Geometry check sheet. Reference: the model listing, model coordinates, mm. A direction names the side the tool comes from. Round coordinates to 2 decimals unless told otherwise and drop trailing zeros. Loops run counter-clockwise (first coordinate to the right, second up) from the corner with the lowest first, then second, coordinate; pieces in that order, holes last. Notation, with made-up numbers: (69.5, 23.5) -> (121.5, 23.5) arc R23 cw to (121.5, 44.5) -> close; hole circle Ø8 at (-21, -23). An arc over 180 degrees is marked (long way). Use a Markdown table: item, result. Add a question column.
Q1. Gauge pin test, flat ends, axial feed: P1, Ø3, axis at x = 8, z = -38, coming from the +Y side; P2, Ø0.8, axis at y = 3.5, z = 34.5, coming from the -X side. Record the tip position at first contact, or that the pin passes through.
Q2. Release check for a two-part mould opening along Y. For faces 3 (the face through (22, 0, -1)), 4 (the face through (44.034, 4.8, 37.675)), 5 (the face through (25, 2, 50)), 6 (the face through (44.034, 4.8, -37.325)) record: released by +Y, released by -Y, zero draft, split by the parting line, or undercut.
Q3. Set-up check for faces 1 (the face through (44, 3, -25)), 2 (the face through (25, 2, -50)): record each of +Z, -Z, +X, -X, +Y, -Y from which the full face is reachable in a straight line by a thin tool's end or side.
Q4. Material ranges on L1, parallel to Y at x = 43.08, z = -39.5; L2, parallel to X at y = 4.5, z = -37.5; L3, parallel to Y at x = 34, z = -24.5, recorded low to high.
Q5. Sectioned sample at D-D, the plane z = 10.5. Enter the section's corners in (x, y).
Q6. Sectioned sample at B-B, the plane y = 1.75. Enter the section's corners in (x, z).
Q7. Sectioned sample at C-C, the plane x = 37. Enter the section's corners in (y, z), then the cut area to 3 significant figures.
Q8. Sectioned sample at A-A, the plane z = -31. Enter the section's corners in (x, y).
Autodesk Inventor part; units mm, degrees
ref_plane "YZ Plane" through (0, 0, 0) normal (1, 0, 0) x (0, 1, 0)
ref_plane "XZ Plane" through (0, 0, 0) normal (0, 1, 0) x (-1, 0, 0)
ref_plane "XY Plane" through (0, 0, 0) normal (0, 0, 1) x (1, 0, 0)
sketch "Эскиз2" plane through (0, 0, 0) normal (0, 0, 1) x (1, 0, 0)
  line L0 (0, 0) -> (45, 0)
  line L1 (45, 0) -> (45, 3)
  line L2 (45, 3) -> (0, 3)
  line L3 (0, 3) -> (0, 0)
  dimension "d14" = 45
  dimension "d15" = 3
extrude "Выдавливание2" add sketch "Эскиз2" along normal mid plane 100
fillet "Сопряжение1" radius 4 2 edges at (0, 1.5, 50) (0, 1.5, -50)
sketch "Эскиз5" plane through (45, 3, 50) normal (0, 1, 0) x (1, 0, 0)
  line L0 (0, 100) -> (0, 0)
  line L1 (0, 0) -> (-41, 0)
  line L2 (0, 100) -> (-3.42, 100)
  line L3 (-3.42, 100) -> (-3.42, 0)
  line L4 (-3.42, 0) -> (0, 0)
  line L5 (0, 0) -> (0, 100)
  point P0 (-45, 50)
  dimension "d25" = 3.42
extrude "Выдавливание4" add sketch "Эскиз5" along normal blind 3
sketch "Эскиз6" plane through (0, 0, 50) normal (0, 0, 1) x (1, 0, 0)
  circle A0 centre (43.08, 4.5) radius 1
  line L0 (41.58, 6) -> (45, 6)
  line L1 (41.58, 3) -> (41.58, 6)
  point P0 (0, 0)
  dimension "d28" = 2
  dimension "d29" = 1.5
  dimension "d30" = 1.5
extrude "Выдавливание5" cut sketch "Эскиз6" against normal through all
sketch "Эскиз7" plane through (45, 6, 50) normal (0, 1, 0) x (1, 0, 0)
  line L0 (-3.42, 100) -> (-3.42, 0)
  line L1 (0, 0) -> (0, 100)
  line L2 (-3.42, 25) -> (0, 25)
  line L3 (0, 25) -> (0, 75)
  line L4 (0, 75) -> (-3.42, 75)
  line L5 (-3.42, 75) -> (-3.42, 25)
  line L6 (-3.42, 0) -> (-41, 0)
  point P0 (-45, 50)
  point P1 (-3.42, 75)
  point P2 (0, 25)
  dimension "d33" = 50
  dimension "d34" = 25
extrude "Выдавливание6" cut sketch "Эскиз7" against normal blind 3
fillet "Сопряжение2" radius 1.5 4 edges at (45, 6, 37.5) (41.58, 6, 37.5) (45, 6, -37.5) (41.58, 6, -37.5)
sketch "Эскиз8" plane through (41.58, 3, -25) normal (0, 0, 1) x (1, 0, 0)
  line L0 (3.42, -3) -> (3.42, 1.5)
  line L1 (0, 0.9343) -> (3.42, -3)
  line L2 (3.42, -3) -> (-37.58, -3)
  line L3 (0, 0) -> (0, 1.5)
  line L4 (0, 0.9343) -> (3.42, 0.9343)
  point P0 (-41.58, -3)
  dimension "d38" = 49
extrude "Выдавливание7" cut sketch "Эскиз8" along normal up to surface (50 mm away)
properties part number "Cover"
Values:
| question | item | result |
|---|---|---|
| 1 | P1 | y = 3 |
| 1 | P2 | x = 41.58 |
| 2 | face 3 | released by -Y |
| 2 | face 4 | undercut |
| 2 | face 5 | zero draft |
| 2 | face 6 | undercut |
| 3 | face 1 | +X, +Y |
| 3 | face 2 | -Z, +X, -X, +Y, -Y |
| 4 | L1 | 0 to 3.5, 5.5 to 6 |
| 4 | L2 | 41.58 to 42.08, 44.08 to 45 |
| 4 | L3 | 0 to 3 |
| 5 | outline | (0, 0) -> (45, 0) -> (42.39, 3) -> (0, 3) -> close |
| 6 | outline | (0, -46) arc R4 ccw to (4, -50) -> (45, -50) -> (45, -25) -> (43.48, -25) -> (43.48, 25) -> (45, 25) -> (45, 50) -> (4, 50) arc R4 ccw to (0, 46) -> close |
| 7 | outline | (0, -50) -> (3, -50) -> (3, 50) -> (0, 50) -> close |
| 7 | area | 300 mm^2 |
| 8 | outline | (0, 0) -> (45, 0) -> (45, 4.5) arc R1.5 ccw to (43.5, 6) -> (43.08, 6) arc R1.5 ccw to (41.58, 4.5) -> (41.58, 3) -> (0, 3) -> close; hole circle Ø2 at (43.08, 4.5) |
